Geometry: final body of the model. Coordinates: model frame, mm. A direction names the side the tool comes from. Round coordinates to 2 decimals unless told otherwise and drop trailing zeros. Order: outer loops, then holes, each group sorted by start corner. A loop starts at its lowest first (then second) coordinate and runs counter-clockwise, first axis right, second up. Notation, with made-up numbers: M -14,48 L 40,48 A28 ccw 40,74 Z; hole C -9.5,86 d8. An arc over 180 degrees is marked long. Return JSON: item names as keys, results as strings. Group by question number.
Q1. Cut plane A-A on x = -4.5. Output: boundary loops of the cut face in (y, z), and give its area (3 significant figures).
Q2. Contact query for flat-ended pins moving along their axis: pin 1 (4 mm diameter, centred on x = 12.5, z = -5, fed in from +Y); pin 2 (4.5 mm diameter, centred on x = -5, z = -0.5, fed in from -Y); pin 3 (2 mm diameter, centred on x = 2, z = -6, fed in from +Y); pin 4 (3 mm diameter, centred on x = -2, z = 3.5, fed in from -Y). Output: stop coordinate, or through.
Q3. Cut plane B-B on x = 31. Output: boundary loops of the cut face in (y, z), and give its area (3 significant figures).
Q4. Access query for faces 1 (the face through (0, 2, -7)), 2 (the face through (35, 0, 0)), 3 (the face through (-5.167, 2.535, 4.31)). Directions: +Z, -Z, +X, -X, +Y, -Y. A direction counts if a zero-diameter tool reaches every point of the face in a straight line with its end or side. Return the directions, or none.
Q5. Ray query, probe 1 along X at (y, z) = (3.25, 7.5); probe 2 along Y at (x, z) = (26.5, 0.25); probe 3 along Z at (x, y) = (31.5, 5.25). Return the intervals inside material, ascending.
Autodesk Inventor part; units mm, degrees
ref_plane "Work Plane1" through (29, 0, 0) normal (0, -1, 0) x (1, 0, 0)
ref_plane "YZ Plane" through (0, 0, 0) normal (1, 0, 0) x (0, 1, 0)
ref_plane "XZ Plane" through (0, 0, 0) normal (0, 1, 0) x (-1, 0, 0)
sketch "Sketch1" plane through (0, 0, 0) normal (0, 0, 1) x (1, 0, 0)
  line L0 (0.6333, 0) -> (35, 0)
  line L1 (35, 0) -> (35, 7)
  line L2 (35, 7) -> (6, 7)
  line L3 (6, 7) -> (4.773, 7)
  line L4 (4.773, 7) -> (0, 7)
  line L5 (0, 7) -> (0, 10.5)
  line L6 (0, 10.5) -> (-8, 10.5)
  line L7 (-8, 10.5) -> (-8, 5.7735)
  line L8 (-8, 5.7735) -> (-2.7, 5.7735)
  line L9 (-2.7, 5.7735) -> (0.6333, 0)
  line L10 (-16.6, 0) -> (43.6, 0)
  line L11 (0, -2.1) -> (0, 12.6)
  line L12 (6, 7) -> (0, 7) construction
  dimension "d1" = 29
  dimension "d2" = 1.227
  dimension "d3" = 8
  dimension "d4" = 5.3
  dimension "d5" = 60
  dimension "d6" = 14
  dimension "d7" = 14
  dimension "d8" = 11.547
  dimension "d9" = 21
  dimension "d26" = 35
revolve "Body" add sketch "Sketch1" angle 360 about axis through (0.6333, 0, 0) along (1, 0, 0) contours L9 L11 L4 L3 L2 L1 L0 | L9 L8 L7 L6 L5 L11
sketch "Sketch2" plane through (-8, 0, 0) normal (-1, 0, 0) x (0, 0, 1)
  circle A0 centre (0, 0) radius 5.7735
  line L0 (0, -14.7) -> (0, 14.7)
  line L1 (-14.7, 0) -> (14.7, 0)
  line L2 (5.7735, 0) -> (2.8868, -5)
  line L3 (2.8868, -5) -> (-2.8868, -5)
  line L4 (-2.8868, -5) -> (-5.7735, 0)
  line L5 (-5.7735, 0) -> (-2.8868, 5)
  line L6 (-2.8868, 5) -> (2.8868, 5)
  line L7 (2.8868, 5) -> (5.7735, 0)
extrude "Slot" add sketch "Sketch2" against normal up to next contours L7 A0 | A0 L2 | L6 L0 A0 | A0 L0 L3 | L0 L6 A0 | A0 L3 L0 | L4 A0 | A0 L5
fillet "Fillet1" radius 1.4 1 edges at (-8, -10.5, 0)
thread "Thread"
chamfer "Chamfer1" distance 1.2269 distance2 1.2269 1 edges at (35, -7, 0) measured on face at (35, -0.3293, 1.9203)
ref_plane "Work Plane1" through (29, 0, 0) normal (0, -1, 0) x (1, 0, 0)
fillet "Fillet2" radius 0.1 1 edges at (0, -7, 0)
equation "\"d1\" = GEL"
equation "\"d3\" = KOH"
equation "\"d4\" = INTI"
equation "\"d6\" = GD"
equation "\"d7\" = BDM"
equation "\"d8\" = 1.1547 * SW"
equation "\"d9\" = KOD"
equation "\"d26\" = NLG"
equation "\"d30\" = R"
equation "\"d17\" = RR"
equation "\"d13\" = GEL"
equation "\"d15\" = -0.5 * SPD + 0.5 * GD"
equation "\"d16\" = GUL"
equation "\"GD\" = NND"
equation "\"NLG\" = 35"
equation "\"GEL\" = 29"
equation "\"KOD\" = 21"
equation "\"KOH\" = 8"
equation "\"INTI\" = 5.3"
equation "\"GAL\" = 0.61345 * PTC"
equation "\"GUL\" = 0.61345 * PTC"
equation "\"BDM\" = NND"
equation "\"RR\" = 1.4"
equation "\"SPD\" = NND - 1.2269 * PTC"
equation "\"R\" = 0.1"
equation "\"TOA\" = 30deg"
equation "\"GD1\" = THREADDIA - 1.2269 * PTC"
equation "\"THREADDIA\" = 14"
equation "\"FAWI\" = 45deg"
equation "\"ANG\" = 120deg"
equation "\"PTC\" = 2"
equation "\"NND\" = 14"
equation "\"E0\" = 1.155 * SW"
properties part number "DIN 7984 - M14 x 35" material "Steel, Mild"
Result sheet:
{
 "1": {"outline": "C 0,0 d21; hole M -5,-2.89 L 0,-5.77 L 5,-2.89 L 5,2.89 L 0,5.77 L -5,2.89 Z", "area": "260 mm²"},
 "2": {"pin 1": "stops at y = 6.32", "pin 2": "stops at y = -10.5", "pin 3": "stops at y = 4.9", "pin 4": "stops at y = -10.31"},
 "3": {"outline": "C 0,0 d14", "area": "154 mm²"},
 "4": {"face 1": "+X", "face 2": "+Z, -Z, +X, +Y, -Y", "face 3": "-X"},
 "5": {"probe 1": "x = -8 to 0", "probe 2": "y = -7 to 7", "probe 3": "z = -4.63 to 4.63"}
}
